Input: part model. Units: mm. Frame: model coordinates. Round coordinates to 2 decimals unless told otherwise and drop trailing zeros. Order: outer loops, then holes, each group sorted by start corner. A loop starts at its lowest first (then second) coordinate and runs counter-clockwise, first axis right, second up. Notation, with made-up numbers: (16, -28.5) -> (42, -28.5) arc R16 cw to (42, -16.5) -> close; hole circle Ø9 at (6.5, 47.25). An arc over 180 degrees is marked (long way). Use a Markdown table: item, result.
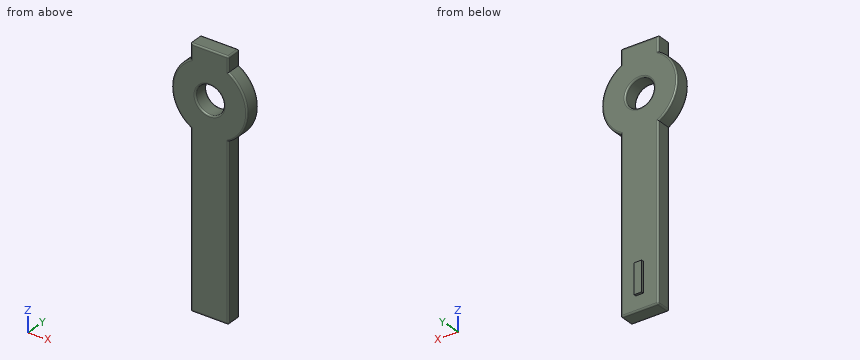
from build123d import *

# Parameters (mm, degrees)
SKETCH_1_R      = 1.875
EXTRUDE_1_DEPTH = 2
FILLET_1_R      = 0.2
SKETCH_2_W      = 1
SKETCH_2_H      = 4
EXTRUDE_2_DEPTH = 0.32


with BuildPart() as part:
    # 草图1 → 凸台-拉伸1 (new body)
    with BuildSketch(Plane(origin=(0, 0, 0), x_dir=(1, 0, 0), z_dir=(0, 1, 0))):
        with BuildLine():
            Line((2.5, 27.330127019), (-2.5, 27.330127019))
            Line((-2.5, 27.330127019), (-2.5, 4.330127019))
            ThreePointArc((-2.5, 4.330127019), (-5, 0), (-2.5, -4.330127019))
            Line((-2.5, -4.330127019), (-2.5, -6.330127019))
            Line((-2.5, -6.330127019), (2.5, -6.330127019))
            Line((2.5, -6.330127019), (2.5, -4.330127019))
            ThreePointArc((2.5, -4.330127019), (5, 0), (2.5, 4.330127019))
            Line((2.5, 4.330127019), (2.5, 27.330127019))
        make_face()
        Circle(SKETCH_1_R, mode=Mode.SUBTRACT)
    extrude(amount=EXTRUDE_1_DEPTH)

    # 圆角1
    fillet_1_edges = [part.edges().sort_by_distance(p)[0] for p in [
        (-1.875, 0, 0),
        (2.5, 2, -15.830127019),
        (2.5, 0, 5.330127019),
        (0, 0, 6.330127019),
        (-2.5, 0, 5.330127019),
        (-5, 0, 0),
        (-2.5, 0, -15.830127019),
        (0, 0, -27.330127019),
        (2.5, 0, -15.830127019),
        (5, 0, 0),
        (0, 2, -27.330127019),
        (2.5, 1, 6.330127019),
        (-2.5, 1, -27.330127019),
        (2.5, 1, -27.330127019),
        (-2.5, 2, -15.830127019),
        (-5, 2, 0),
        (-2.5, 2, 5.330127019),
        (0, 2, 6.330127019),
        (2.5, 2, 5.330127019),
        (-1.875, 2, 0),
        (5, 2, 0),
    ]]
    fillet(fillet_1_edges, radius=FILLET_1_R)

    # 草图2 → 凸台-拉伸2 (add)
    with BuildSketch(Plane(origin=(0, 2, 0), x_dir=(1, 0, 0), z_dir=(0, 1, 0))):
        with Locations((0, 23.330127019)):
            Rectangle(SKETCH_2_W, SKETCH_2_H)
    extrude(amount=EXTRUDE_2_DEPTH)


solid = part.part
1) Cut plane B-B on y = 0.55. Return loops of the section in (x, z) (3 decimals).
Results found:
| item | result |
|---|---|
| outline | (-2.5, -27.13) arc R0.2 ccw to (-2.3, -27.33) -> (2.3, -27.33) arc R0.2 ccw to (2.5, -27.13) -> (2.5, -4.33) arc R5 ccw to (2.5, 4.33) -> (2.5, 6.13) arc R0.2 ccw to (2.3, 6.33) -> (-2.5, 6.33) -> (-2.5, 4.33) arc R5 ccw to (-2.5, -4.33) -> close; hole circle Ø3.75 at (0, 0) |
2) Line query: L1, parallel to Z at x = 0, y = 0.75 (3 decimals); L2, parallel to Y at x = 0.75, z = -7; L3, parallel to X at y = 0.65, z = -5.5. Output: solid intervals per line, ascending. Write a range as [from, to].
Results found:
| item | result |
|---|---|
| L1 | z = [-27.33, -1.875], [1.875, 6.33] |
| L2 | y = [0, 2] |
| L3 | x = [-2.5, 2.5] |
3) Cut plane D-D on z = -11.5. Return loops of the section in (x, y).
Results found:
| item | result |
|---|---|
| outline | (-2.5, 0.2) arc R0.2 ccw to (-2.3, 0) -> (2.3, 0) arc R0.2 ccw to (2.5, 0.2) -> (2.5, 1.8) arc R0.2 ccw to (2.3, 2) -> (-2.3, 2) arc R0.2 ccw to (-2.5, 1.8) -> close |
4) Cut plane A-A on z = 0. Return loops of the section in (x, y) (3 decimals).
Results found:
| item | result |
|---|---|
| outline | (-5, 0.2) arc R0.2 ccw to (-4.8, 0) -> (-2.075, 0) arc R0.2 ccw to (-1.875, 0.2) -> (-1.875, 1.8) arc R0.2 ccw to (-2.075, 2) -> (-4.8, 2) arc R0.2 ccw to (-5, 1.8) -> close; (1.875, 0.2) arc R0.2 ccw to (2.075, 0) -> (4.8, 0) arc R0.2 ccw to (5, 0.2) -> (5, 1.8) arc R0.2 ccw to (4.8, 2) -> (2.075, 2) arc R0.2 ccw to (1.875, 1.8) -> close |
5) Pin query (flat end, axial travel): pin 1 Ø3 at (x, z) = (1, -13.5) entering from +Y; pin 2 Ø0.8 at (y, z) = (1.5, -11.5) entering from -X; pin 3 Ø1 at (y, z) = (1.5, 1.5) entering from +X. Return the tip coordinate at first contact, or that it passes through.
Results found:
| item | result |
|---|---|
| pin 1 | stops at y = 2 |
| pin 2 | stops at x = -2.5 |
| pin 3 | stops at x = 4.9 |
6) Cut plane C-C on x = 0. Return loops of the section in (y, z) (3 decimals), and give its area (3 significant figures).
Results found:
| item | result |
|---|---|
| outline | (0, -27.13) arc R0.2 ccw to (0.2, -27.33) -> (1.8, -27.33) arc R0.2 ccw to (2, -27.13) -> (2, -25.33) -> (2.32, -25.33) -> (2.32, -21.33) -> (2, -21.33) -> (2, -2.075) arc R0.2 ccw to (1.8, -1.875) -> (0.2, -1.875) arc R0.2 ccw to (0, -2.075) -> close; (0, 2.075) arc R0.2 ccw to (0.2, 1.875) -> (1.8, 1.875) arc R0.2 ccw to (2, 2.075) -> (2, 6.13) arc R0.2 ccw to (1.8, 6.33) -> (0.2, 6.33) arc R0.2 ccw to (0, 6.13) -> close |
| area | 61.0 mm² |
